Verification items for the finished model (mm, model axes). A direction names the side the tool comes from. Give positions to 0.01 mm unless a question says otherwise; leave off trailing zeros. Order: outer loops, then holes, each group sorted by start corner. A loop starts at its lowest first (then second) coordinate and runs counter-clockwise, first axis right, second up. Notation, with made-up numbers: (36, 18) -> (48, 18) arc R17 ccw to (48, 44) -> close; hole circle Ø11 at (-29.75, 51). An arc over 180 degrees is marked (long way). One line per question, with ' | ' between items. Start each with the question number.
Q1. Mould release check, pull along X, two halves, no side actions. Record for faces 1 (the cylindrical face through (-24.43, 0.35, 1.6)), 2 (the flat face through (18.329, 0, 19)), 3 (the flat face through (14.329, 0, 19)), 4 (the flat face through (24, 0, 31)): released by +X, released by -X, zero draft, split by the parting line, or undercut.
Q2. Access from +Z, -Z, +X, -X, +Y, -Y to the whole of each face (thin tool, end or side, straight path). Record for faces 5 (the flat face through (-24, 0, 31)), 6 (the flat face through (6.329, 0, 19)).
Q3. Go/stop test with flat-tipped pins: pin 1 (3 mm diameter, centred on x = 13.5, y = 15.5, fed in from -Z); pin 2 (0.6 mm diameter, centred on x = -8, y = -9, fed in from +Z). Record where each tip stops, or that it passes through.
Q4. Section check A-A on z = 25. Give the number of separate pieces and of enclosed holes in the cut face, plus the area to 3 significant figures.
Q5. Section check B-B on x = 13. Record the cut outline in (y, z).
Q6. Material ranges on probe 1 along Z at (x, y) = (5, -4); probe 2 along Z at (x, y) = (-8, -11); probe 3 along X at (y, z) = (-9, 2.5), recorded low to high. Write a range as [from, to].
from build123d import *

# Parameters (mm, degrees)
SKETCH1_R           = 10
BOSS_EXTRUDE1_DEPTH = 1
SKETCH2_W           = 50
SKETCH2_H           = 50
BOSS_EXTRUDE2_DEPTH = 30
SKETCH3_W           = 2
SKETCH3_H           = 50
CUT_EXTRUDE1_DEPTH  = 25
FILLET1_R           = 2


with BuildPart() as part:
    # Sketch1 → Boss-Extrude1 (new body)
    with BuildSketch(Plane.XY):
        Circle(SKETCH1_R)
    extrude(amount=BOSS_EXTRUDE1_DEPTH)

    # Sketch2 → Boss-Extrude2 (add)
    with BuildSketch(Plane.XY.offset(1)):
        Rectangle(SKETCH2_W, SKETCH2_H)
    extrude(amount=BOSS_EXTRUDE2_DEPTH)

    # Sketch3 → Cut-Extrude1 (cut)
    with BuildSketch(Plane.XY.offset(31)):
        with Locations((-22.6705156, 0)):
            Rectangle(SKETCH3_W, SKETCH3_H)
        with Locations((-19.6705156, 0)):
            Rectangle(SKETCH3_W, SKETCH3_H)
        with Locations((-16.6705156, 0)):
            Rectangle(SKETCH3_W, SKETCH3_H)
        with Locations((-13.6705156, 0)):
            Rectangle(SKETCH3_W, SKETCH3_H)
        with Locations((-10.6705156, 0)):
            Rectangle(SKETCH3_W, SKETCH3_H)
        with Locations((-7.6705156, 0)):
            Rectangle(SKETCH3_W, SKETCH3_H)
        with Locations((-4.6705156, 0)):
            Rectangle(SKETCH3_W, SKETCH3_H)
        with Locations((-1.6705156, 0)):
            Rectangle(SKETCH3_W, SKETCH3_H)
        with Locations((1.3294844, 0)):
            Rectangle(SKETCH3_W, SKETCH3_H)
        with Locations((4.3294844, 0)):
            Rectangle(SKETCH3_W, SKETCH3_H)
        with Locations((7.3294844, 0)):
            Rectangle(SKETCH3_W, SKETCH3_H)
        with Locations((10.3294844, 0)):
            Rectangle(SKETCH3_W, SKETCH3_H)
        with Locations((13.3294844, 0)):
            Rectangle(SKETCH3_W, SKETCH3_H)
        with Locations((16.3294844, 0)):
            Rectangle(SKETCH3_W, SKETCH3_H)
        with Locations((19.3294844, 0)):
            Rectangle(SKETCH3_W, SKETCH3_H)
        with Locations((22.3294844, 0)):
            Rectangle(SKETCH3_W, SKETCH3_H)
    extrude(amount=-CUT_EXTRUDE1_DEPTH, mode=Mode.SUBTRACT)

    # Fillet1
    fillet1_edges = [part.edges().sort_by_distance(p)[0] for p in [
        (25, 0, 1),
        (-25, 0, 1),
    ]]
    fillet(fillet1_edges, radius=FILLET1_R)


solid = part.part
Filled in:
1) face 1: released by -X | face 2: undercut | face 3: undercut | face 4: zero draft
2) face 5: +Z, +X, -X, +Y, -Y | face 6: +Z, +Y, -Y
3) pin 1: z = 1 | pin 2: z = 6
4) separate pieces: 17 | enclosed holes: 0 | area: 900 mm²
5) outline: (-25, 1) -> (25, 1) -> (25, 6) -> (-25, 6) -> close
6) probe 1: [0, 6] | probe 2: [1, 6] | probe 3: [-24.94, 24.94]
